from build123d import *

# Parameters (mm, degrees)
SKETCH1_W           = 56
SKETCH1_H           = 88
BOSS_EXTRUDE1_DEPTH = 44
SKETCH1_3_R         = 15
BOSS_EXTRUDE2_DEPTH = 83
SKETCH2_W           = 82
SKETCH2_H           = 106
CUT_EXTRUDE1_DEPTH  = 83
CUT_EXTRUDE2_DEPTH  = 56
SKETCH3_4_R         = 25
CUT_EXTRUDE3_DEPTH  = 196
SKETCH5_R           = 25
CUT_EXTRUDE6_DEPTH  = 246


with BuildPart() as part:
    # Sketch1 → Boss-Extrude1 (new, symmetric)
    with BuildSketch(Plane.XY):
        Rectangle(SKETCH1_W, SKETCH1_H)
    extrude(amount=BOSS_EXTRUDE1_DEPTH, both=True)

    # Sketch1_3 → Boss-Extrude2 (add, symmetric)
    with BuildSketch(Plane.XY):
        with BuildLine():
            Line((-58, 44), (-102, 38))
            ThreePointArc((-102, 38), (-140, 0), (-102, -38))
            Line((-102, -38), (-58, -44))
            Line((-58, -44), (-28, -44))
            Line((-28, -44), (-28, 44))
            Line((-28, 44), (-58, 44))
        make_face()
        with Locations((-102, 0)):
            Circle(SKETCH1_3_R, mode=Mode.SUBTRACT)
    extrude(amount=BOSS_EXTRUDE2_DEPTH, both=True)

    # Sketch2 → Cut-Extrude1 (cut, symmetric)
    with BuildSketch(Plane(origin=(0, 0, 0), x_dir=(1, 0, 0), z_dir=(0, 1, 0))):
        with Locations((-99, 0)):
            Rectangle(SKETCH2_W, SKETCH2_H)
    extrude(amount=CUT_EXTRUDE1_DEPTH, both=True, mode=Mode.SUBTRACT)

    # Sketch3 → Cut-Extrude2 (cut)
    with BuildSketch(Plane(origin=(28, 0, 0), x_dir=(0, 0, -1), z_dir=(1, 0, 0))):
        with BuildLine():
            Line((-44, 44), (-44, 0))
            ThreePointArc((-44, 0), (-31.112698372, 31.112698372), (0, 44))
            Line((0, 44), (-44, 44))
        make_face()
        with BuildLine():
            Line((44, 44), (0, 44))
            ThreePointArc((0, 44), (31.112698372, 31.112698372), (44, 0))
            Line((44, 0), (44, 44))
        make_face()
        with BuildLine():
            ThreePointArc((44, 0), (31.112698372, -31.112698372), (0, -44))
            Line((0, -44), (44, -44))
            Line((44, -44), (44, 0))
        make_face()
        with BuildLine():
            ThreePointArc((0, -44), (-31.112698372, -31.112698372), (-44, 0))
            Line((-44, 0), (-44, -44))
            Line((-44, -44), (0, -44))
        make_face()
    extrude(amount=-CUT_EXTRUDE2_DEPTH, mode=Mode.SUBTRACT)

    # Sketch3_4 → Cut-Extrude3 (cut)
    with BuildSketch(Plane(origin=(28, 0, 0), x_dir=(0, 0, -1), z_dir=(1, 0, 0))):
        Circle(SKETCH3_4_R)
    extrude(amount=-CUT_EXTRUDE3_DEPTH, mode=Mode.SUBTRACT)

    # Sketch5 → Cut-Extrude6 (cut)
    with BuildSketch(Plane(origin=(28, 0, 0), x_dir=(0, 0, -1), z_dir=(1, 0, 0))):
        Circle(SKETCH5_R)
        with BuildLine():
            Line((8, 30), (8, 23.685438565))
            ThreePointArc((8, 23.685438565), (0, 25), (-8, 23.685438565))
            Line((-8, 23.685438565), (-8, 30))
            Line((-8, 30), (8, 30))
        make_face()
    extrude(amount=-CUT_EXTRUDE6_DEPTH, mode=Mode.SUBTRACT)


solid = part.part
The listing builds one solid part. Answer for the finished solid, in the listing's coordinates (mm). A direction names the side the tool comes from. Give positions to 0.01 mm unless a question says otherwise; leave off trailing zeros. Write each loop counter-clockwise with the first axis right and the second up, starting at its lowest first coordinate (ties: lowest second). Pieces come first, ordered by that corner, then holes.
1) Section D-D (z = 12.5) is taken. Write down the section's boundary in (x, y), and give its area (3 significant figures).
2) Section C-C (x = -111) is taken. Write down the section's boundary in (y, z).
3) Given P1, Ø1.5, axis at y = -15, z = -65.5, coming from the +X side; P2, Ø8, axis at x = -13, z = 44, coming from the -Y side; P3, Ø7, axis at x = -2, y = 26.5, coming from the -Z side, each flat-ended and moving along its own axis, determine where each tip first touches the part or whether it passes through.
4) Find the intervals of material crossed by L1, parallel to Z at x = -40, y = 0; L2, parallel to X at y = 0, z = -62; L3, parallel to Z at x = -77, y = 15, in increasing order.
5) For a pull along Z with two mould halves and no side action, classify faces 4 (the face through (-90, 10, 53)), 5 (the face through (-72, 1, 83)), 6 (the face through (-80, -41, 68)) as pulls with the +Z half, pulls with the -Z half, needs draft (parallel to the pull), parting line crosses it, or undercut.
6) A tool of negligible diameter and unlimited length cuts with its end or side. For faces 1 (the face through (-139.99, 0.84, 68.21)), 2 (the face through (-90, 10, -53)), 3 (the face through (-14, 27, 8)), from which of +Z, -Z, +X, -X, +Y, -Y can it reach the whole face along a straight path? Write none if from no direction.
7) Section A-A (x = -9) is taken. Write down the section's boundary in (y, z).
8) Section B-B (y = 9.5) is taken. Write down the section's boundary in (x, z).
Response:
1. outline: (-58, -44) - (-28, -44) - (-28, -42.19) - (28, -42.19) - (28, -21.65) - (-58, -21.65) - close; (-58, 21.65) - (28, 21.65) - (28, 42.19) - (-28, 42.19) - (-28, 44) - (-58, 44) - close
1. area: 3,640 mm2
2. outline: (-36.92, -83) - (-12, -83) - (-12, -53) - (-36.92, -53) - close; (-36.92, 53) - (-12, 53) - (-12, 83) - (-36.92, 83) - close; (12, -83) - (36.92, -83) - (36.92, -53) - (12, -53) - close; (12, 53) - (36.92, 53) - (36.92, 83) - (12, 83) - close
3. P1: stops at x = -28
3. P2: stops at y = -18.33
3. P3: stops at z = -37.51
4. L1: z = -83 to -25, 25 to 83
4. L2: x = -140 to -117, -87 to -28
4. L3: z = -83 to -53, 53 to 83
5. face 4: undercut
5. face 5: pulls with the +Z half
5. face 6: needs draft
6. face 1: +Z, -Z, -X
6. face 2: -X, +Y, -Y
6. face 3: +X, -X
7. outline: circle Ø88 at (0, 0); hole (23.69, -8) - (30, -8) - (30, 8) - (23.69, 8) arc R25 ccw (long way) to start
8. outline: (-138.79, -83) - (-113.61, -83) - (-113.61, -53) - (-138.79, -53) - close; (-138.79, 53) - (-113.61, 53) - (-113.61, 83) - (-138.79, 83) - close; (-90.39, -83) - (-28, -83) - (-28, -42.96) - (28, -42.96) - (28, -23.12) - (-58, -23.12) - (-58, -53) - (-90.39, -53) - close; (-90.39, 53) - (-58, 53) - (-58, 23.12) - (28, 23.12) - (28, 42.96) - (-28, 42.96) - (-28, 83) - (-90.39, 83) - close
